The listing builds one solid part. Answer for the finished solid, in the listing's coordinates (mm). Face numbers are marked on the shaded views. A direction names the side the tool comes from. Round coordinates to 2 decimals unless told otherwise and drop trailing zeros. Loops run counter-clockwise (first coordinate to the right, second up) from the corner with the lowest first, then second, coordinate; pieces in that order, holes last. Notation, with made-up numbers: (29.25, 53.5) - (35.25, 53.5) arc R7 ccw to (35.25, 57.5) - close; hole circle Ø10 at (10.25, 24). An arc over 180 degrees is marked (long way). Write item = value, one per line. Start each with the question number.
1) Given pin 1 Ø2 at (x, z) = (14, 1) entering from +Y; pin 2 Ø1.5 at (x, z) = (-12, 1) entering from +Y; pin 3 Ø1.5 at (y, z) = (4.5, 0.5) entering from -X; pin 4 Ø3 at (y, z) = (19, -1.5) entering from +X (3 decimals), each flat-ended and moving along its own axis, determine where each tip first touches the part or whether it passes through.
2) For a pull along Y with two mould halves and no side action, classify the marked faces 4, 5 and 6 as released by +Y, released by -Y, zero draft, split by the parting line, or undercut.
3) Section B-B, the plane x = 0.05 is taken. Determine the outline of the cut face in (y, z).
4) Section A-A, the plane x = 14 is taken. Determine the outline of the cut face in (y, z), and give its area (4 significant figures).
5) Section C-C, the plane z = 3.75 is taken. Determine the outline of the cut face in (x, y) (3 decimals), and give its area (3 significant figures).
6) A tool of negligible diameter and unlimited length cuts with its end or side. For the marked faces 1, 2 and 3, from which of +Z, -Z, +X, -X, +Y, -Y can it reach the whole face along a straight path? Write none if from no direction.
7) Section D-D, the plane y = 4.25 is taken. Determine the outline of the cut face in (x, z).
8) Straight lines are drawn through the part: line 1 along Z through (x, y) = (-14, 17); line 2 along Y through (x, z) = (-3, -0.75); line 3 along X through (y, z) = (16.8, 0). For each, find the intervals that lie inside material, in ascending order.
from build123d import *

# Parameters (mm, degrees)
SKETCH_1_W          = 23.8
SKETCH_1_H          = 11.5
EXTRUDE_1_DEPTH     = 21.65
EXTRUDE_START       = -16.3
SKETCH_2_W          = 32.05
SKETCH_2_H          = 11.5
EXTRUDE_2_DEPTH     = 1.5
SKETCH_3_R          = 2.75
SKETCH_3_R_2        = 5.75
EXTRUDE_3_DEPTH     = 4.15
SKETCH_4_R          = 2.5
EXTRUDE_4_DEPTH     = 3.45
CHAMFER_1_SIZE      = 1
CUT_EXTRUDE_1_REACH = 26.631
SKETCH_5_R          = 1


with BuildPart() as part:
    # Sketch 1 → Extrude 1 (new body)
    with BuildSketch(Plane(origin=(0, 0, 0), x_dir=(1, 0, 0), z_dir=(0, 1, 0))):
        Rectangle(SKETCH_1_W, SKETCH_1_H)
    extrude(amount=EXTRUDE_1_DEPTH)

    # Sketch 2 → Extrude 2 (add)
    with BuildSketch(Plane.XZ.offset(EXTRUDE_START)):
        Rectangle(SKETCH_2_W, SKETCH_2_H)
    extrude(amount=-EXTRUDE_2_DEPTH)

    # Sketch 3 → Extrude 3 (add)
    with BuildSketch(Plane(origin=(0, 21.65, 0), x_dir=(1, 0, 0), z_dir=(0, 1, 0))):
        with Locations((0.05, 0)):
            Circle(SKETCH_3_R)
        with Locations((-6.15, 0)):
            Circle(SKETCH_3_R_2)
    extrude(amount=EXTRUDE_3_DEPTH)

    # Sketch 4 → Extrude 4 (add)
    with BuildSketch(Plane(origin=(0, 25.8, 0), x_dir=(1, 0, 0), z_dir=(0, 1, 0))):
        with Locations(Location((-6.15, 0, 0), (0, 0, 90))):
            Circle(SKETCH_4_R)
    extrude(amount=EXTRUDE_4_DEPTH)

    # Chamfer 1
    chamfer_1_edges = [part.edges().sort_by_distance(p)[0] for p in [
        (-16.025, 17.05, 5.75),
        (16.025, 17.05, -5.75),
        (-16.025, 17.05, -5.75),
        (16.025, 17.05, 5.75),
    ]]
    chamfer(chamfer_1_edges, length=CHAMFER_1_SIZE)

    # Sketch 5 → Cut-Extrude 1 (cut, up to next)
    with BuildSketch(Plane(origin=(0, 17.8, 0), x_dir=(1, 0, 0), z_dir=(0, 1, 0)), mode=Mode.PRIVATE) as cut_extrude_1_sk1:
        with Locations((14, 0)):
            Circle(SKETCH_5_R)
    cut_extrude_1_tool1 = extrude(cut_extrude_1_sk1.sketch, amount=-CUT_EXTRUDE_1_REACH, mode=Mode.PRIVATE) & part.part
    # Sketch 5 → Cut-Extrude 1 (cut, up to next)
    with BuildSketch(Plane(origin=(0, 17.8, 0), x_dir=(1, 0, 0), z_dir=(0, 1, 0)), mode=Mode.PRIVATE) as cut_extrude_1_sk2:
        with BuildLine():
            Line((16.025, -0.6), (16.025, 0.6))
            Line((16.025, 0.6), (14.8, 0.6))
            ThreePointArc((14.8, 0.6), (14.948683298, 0.316227766), (15, 0))
            ThreePointArc((15, 0), (14.948683298, -0.316227766), (14.8, -0.6))
            Line((14.8, -0.6), (16.025, -0.6))
        make_face()
    cut_extrude_1_tool2 = extrude(cut_extrude_1_sk2.sketch, amount=-CUT_EXTRUDE_1_REACH, mode=Mode.PRIVATE) & part.part
    cut_extrude_1_1 = cut_extrude_1_tool1.solids().sort_by_distance((14, 17.8, 0))[0]
    add(cut_extrude_1_1, mode=Mode.SUBTRACT)
    cut_extrude_1_2 = cut_extrude_1_tool2.solids().sort_by_distance((15.479048, 17.8, 0))[0]
    add(cut_extrude_1_2, mode=Mode.SUBTRACT)
    cut_extrude_1 = cut_extrude_1_1 + cut_extrude_1_2  # Cut-Extrude 1 as one shape, for the pattern or mirror that repeats it

    # Mirror 1: Cut-Extrude 1 across plane
    add(cut_extrude_1.mirror(Plane(origin=(0, 0, 0), x_dir=(0, 0, 1), z_dir=(1, 0, 0))), mode=Mode.SUBTRACT)


solid = part.part
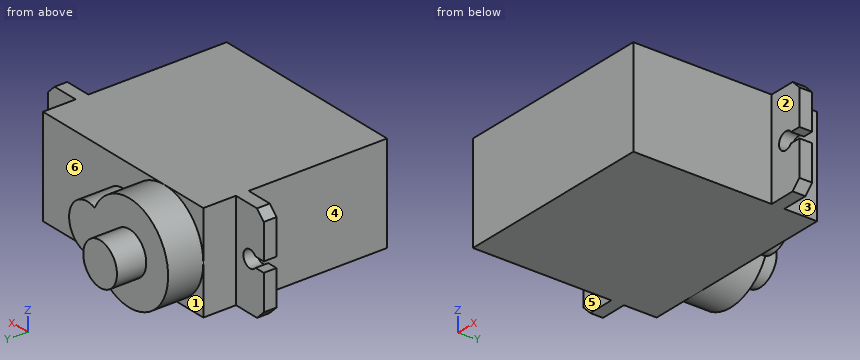
Geometry check:
q1.pin_1 = 17.8
q1.pin_2 = 25.8
q1.pin_3 = -11.9
q1.pin_4 = 16.025
q2.face_4 = zero draft
q2.face_5 = released by -Y
q2.face_6 = released by +Y
q3.outline = (0, -5.75) - (21.65, -5.75) - (21.65, -2.75) - (25.8, -2.75) - (25.8, 2.75) - (21.65, 2.75) - (21.65, 5.75) - (0, 5.75) - close
q4.outline = (16.3, -5.75) - (17.8, -5.75) - (17.8, -1) - (16.3, -1) - close; (16.3, 1) - (17.8, 1) - (17.8, 5.75) - (16.3, 5.75) - close
q4.area = 14.25 mm2
q5.outline = (-16.025, 16.3) - (-11.9, 16.3) - (-11.9, 0) - (11.9, 0) - (11.9, 16.3) - (16.025, 16.3) - (16.025, 17.8) - (11.9, 17.8) - (11.9, 21.65) - (-1.791, 21.65) - (-1.791, 25.8) - (-10.509, 25.8) - (-10.509, 21.65) - (-11.9, 21.65) - (-11.9, 17.8) - (-16.025, 17.8) - close
q5.area = 564 mm2
q6.face_1 = -Z, -X, +Y
q6.face_2 = +Z, -Z, +X, -Y
q6.face_3 = +Z, -Z, +X, +Y
q7.outline = (-11.9, -5.75) - (11.9, -5.75) - (11.9, 5.75) - (-11.9, 5.75) - close
q8.line_1 = -5.75 to -1, 1 to 5.75
q8.line_2 = 0 to 25.8
q8.line_3 = -13 to 13
